```python
from build123d import *

# Parameters (mm, degrees)
SKETCH2_R          = 2.7
CUT_EXTRUDE1_DEPTH = 22


with BuildPart() as part:
    # Sketch1 → Revolve1 (revolve)
    with BuildSketch(Plane.XY):
        Polygon((0, 0), (35, 0), (35, 11.1), (16.4, 11.1), (16.4, 22), (14, 22), (14, 11.1), (9, 11.1), (9, 3.9), (0, 3.9), align=None)
    revolve(axis=Axis((0, 0, 0), (1, 0, 0)))

    # Sketch2 → Cut-Extrude1 (cut, through all)
    with BuildSketch(Plane.ZY.offset(-14)):
        with Locations((0, 17.5)):
            Circle(SKETCH2_R)
        with Locations((15.155444566, -8.75)):
            Circle(SKETCH2_R)
        with Locations((-15.155444566, -8.75)):
            Circle(SKETCH2_R)
    extrude(amount=-CUT_EXTRUDE1_DEPTH, mode=Mode.SUBTRACT)


solid = part.part
```
Model file for the job. Use its own axes, mm. A direction names the side the tool comes from. Give positions to 0.01 mm unless a question says otherwise; leave off trailing zeros. Write each loop counter-clockwise with the first axis right and the second up, starting at its lowest first coordinate (ties: lowest second). Pieces come first, ordered by that corner, then holes. Notation, with made-up numbers: (-30, -39) -> (-1, -39) arc R9 ccw to (-1, -33) -> close; hole circle Ø11 at (-16.75, 37). An arc over 180 degrees is marked (long way). Use CSV: the item, a comma, the result in double quotes. Start each with the question number.
1) Cut at C-C on y = 17.5. List the corners of the cut face in (x, z), plus the area to 3 significant figures.
2) Cut at A-A on z = 0. List the corners of the cut face in (x, y).
3) Tool access for faces 1 (the cylindrical face through (15.183, 20.177, -0.351)), 2 (the cylindrical face through (25.57, 5.97, 9.36)), 3 (the cylindrical face through (11.46, 5.97, 9.36)): list every direction of +Z, -Z, +X, -X, +Y, -Y with a clear straight run to the whole face (end or side of a thin tool).
4) Pin check, flat tips, straight feed: P1, Ø1.5, axis at y = 13.5, z = -3, coming from the -X side; P2, Ø1, axis at x = 25, y = 4, coming from the +Z side; P3, Ø4, axis at x = 17, z = 15.5, coming from the -Y side; P4, Ø22, axis at y = 7.5, z = 2, coming from the -X side. Stop position of each tip, or through.
5) Cut at D-D on y = 0. List the corners of the cut face in (x, z), plus the area to 3 significant figures.
6) Drill centre lines: L1, parallel to X at y = 11.5, z = 11; L2, parallel to Z at x = 15, y = -8; L3, parallel to X at y = 3, z = 7.5. Where is each one in solid material? Low to high.
7) Two-plate mould, pull along Y, no slides. Class faces 4 (the flat face through (16.4, 5.2, 10.1)), 5 (the cylindrical face through (4.44, -2.87, 2.64)), 6 (the cylindrical face through (15.18, -9.78, 17.65)): released by +Y, released by -Y, zero draft, split by the parting line, or undercut.
8) Cut at B-B on y = -8.75. List the corners of the cut face in (x, z), plus the area to 3 significant figures.
Final values:
1,outline,"(14, -13.33) -> (16.4, -13.33) -> (16.4, -2.7) -> (14, -2.7) -> close; (14, 2.7) -> (16.4, 2.7) -> (16.4, 13.33) -> (14, 13.33) -> close"
1,area,"51.0 mm2"
2,outline,"(0, -3.9) -> (9, -3.9) -> (9, -11.1) -> (14, -11.1) -> (14, -22) -> (16.4, -22) -> (16.4, -11.1) -> (35, -11.1) -> (35, 11.1) -> (16.4, 11.1) -> (16.4, 14.8) -> (14, 14.8) -> (14, 11.1) -> (9, 11.1) -> (9, 3.9) -> (0, 3.9) -> close; (14, 20.2) -> (16.4, 20.2) -> (16.4, 22) -> (14, 22) -> close"
3,face 1,"+X, -X"
3,face 2,"+X"
3,face 3,"-X"
4,P1,"stops at x = 14"
4,P2,"stops at z = 10.53"
4,P3,"stops at y = -17.3"
4,P4,"stops at x = 0"
5,outline,"(0, -3.9) -> (9, -3.9) -> (9, -11.1) -> (14, -11.1) -> (14, -22) -> (16.4, -22) -> (16.4, -11.1) -> (35, -11.1) -> (35, 11.1) -> (16.4, 11.1) -> (16.4, 22) -> (14, 22) -> (14, 11.1) -> (9, 11.1) -> (9, 3.9) -> (0, 3.9) -> close"
5,area,"700 mm2"
6,L1,"x = 14 to 16.4"
6,L2,"z = -20.49 to -17.75, -12.56 to 12.56, 17.75 to 20.49"
6,L3,"x = 9 to 35"
7,face 4,"zero draft"
7,face 5,"split by the parting line"
7,face 6,"undercut"
8,outline,"(9, -6.83) -> (14, -6.83) -> (14, -12.46) -> (16.4, -12.46) -> (16.4, -6.83) -> (35, -6.83) -> (35, 6.83) -> (16.4, 6.83) -> (16.4, 12.46) -> (14, 12.46) -> (14, 6.83) -> (9, 6.83) -> close; (14, -20.19) -> (16.4, -20.19) -> (16.4, -17.86) -> (14, -17.86) -> close; (14, 17.86) -> (16.4, 17.86) -> (16.4, 20.19) -> (14, 20.19) -> close"
8,area,"393 mm2"
